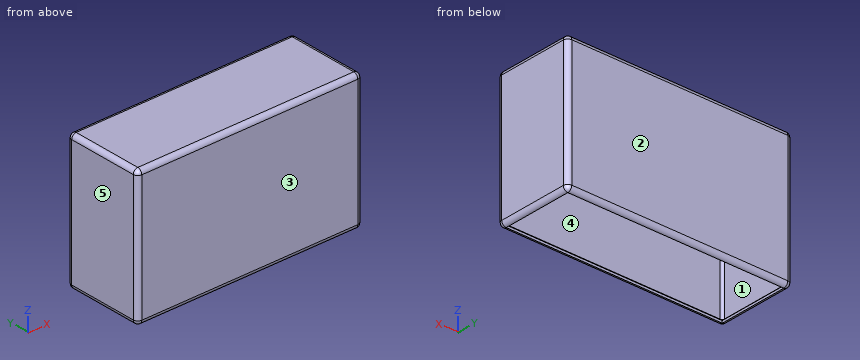
```python
from build123d import *

# Parameters (mm, degrees)
F0_W     = 254
F0_H     = 152.4
F1_DEPTH = 88.9
F2_R     = 5.08
F3_R     = 5.08
F4_R     = 5.08
F5_T     = -2.54


# Not quite as in the source:
# - a shell that OpenCascade refuses in one call is made with other operations: the cavity is built on its own and cut out


with BuildPart() as f1:
    # F0 (on Front) → F1 (new body)
    with BuildSketch(Plane.XZ):
        with Locations((-5.4093236282, -1.1136829853)):
            Rectangle(F0_W, F0_H)
    extrude(amount=F1_DEPTH)

    # F2
    f2_edges = [f1.edges().sort_by_distance(p)[0] for p in [
        (121.590676, -88.9, -1.113683),
        (121.590676, 0, -1.113683),
    ]]
    fillet(f2_edges, radius=F2_R)

    # F3
    f3_edges = [f1.edges().sort_by_distance(p)[0] for p in [
        (-7.949324, -88.9, 75.086317),
        (-7.949324, -88.9, -77.313683),
    ]]
    fillet(f3_edges, radius=F3_R)

    # F4
    f4_edges = [f1.edges().sort_by_distance(p)[0] for p in [
        (-132.409324, 0, -1.113683),
        (-132.409324, -88.9, -1.113683),
    ]]
    fillet(f4_edges, radius=F4_R)

    # F5: a shell. OpenCascade refuses it in one call, so the cavity is built on its own and cut out:
    # the body offset inwards by the wall thickness, plus a prism from it out through each open face.
    f5_core = offset(f1.part, amount=F5_T, mode=Mode.PRIVATE)
    f5_exits = [f5_core.faces().sort_by_distance(p)[0] for p in [
        (-5.409324, -44.45, -74.773683),
    ]]
    add(f5_core, mode=Mode.SUBTRACT)
    extrude(f5_exits, amount=-F5_T, mode=Mode.SUBTRACT)


solid = f1.part
```
Could you check a few things on this model? Use its own coordinates, in mm. Face numbers are marked on the shaded views. A direction names the side the tool comes from. Coordinates: 2 decimals unless noted, no trailing zeros. Order: outer loops, then holes, each group sorted by start corner. A loop starts at its lowest first (then second) coordinate and runs counter-clockwise, first axis right, second up. Notation, with made-up numbers: M 23,-33 L 62,-33 A20 cw 62,-27 Z; hole C 79.25,68.25 d5. An arc over 180 degrees is marked long. Use a Markdown table: item, result. Add a question column.
Q1. Which directions (+Z, -Z, +X, -X, +Y, -Y) give clear straight access to the entire face, cutting with the end or side of a thin tool? Please do the marked faces 1 and 2.
Q2. If I drill on L1, parallel to X at y = -12, z = 61; L2, parallel to Y at x = 3, z = -59; L3, parallel to Z at x = -84.5, y = -64, over which ranges is the centre line in solid material (lowest first)?
Q3. I want a section at A-A on z = -56. List the corners of the cut face in (x, y) for me.
Q4. I want a section at B-B on y = -80. List the corners of the cut face in (x, z) for me.
Q5. I want a section at C-C on x = 100. List the corners of the cut face in (y, z) for me.
Q6. We'd pull the mould along Y, two halves only. Please class the marked faces 3, 4 and 5: pulls with the +Y half, pulls with the -Y half, needs draft (parallel to the pull), parting line crosses it, or undercut.
Q7. I'm going to push flat-ended pins straight in: pin 1 (12 mm diameter, centred on x = -102.5, y = -65, fed in from -Z); pin 2 (0.8 mm diameter, centred on y = -54, z = -76, fed in from -X); pin 3 (2 mm diameter, centred on x = 40.5, z = -76.5, fed in from +Y). Where does each tip first touch, or does it pass through?
Checked values:
| question | item | result |
|---|---|---|
| 1 | face 1 | none |
| 1 | face 2 | +Z, -Z, +X, -X, +Y |
| 2 | L1 | -132.41 to -129.87, 119.05 to 121.59 |
| 2 | L2 | -88.9 to -86.36, -2.54 to 0 |
| 2 | L3 | 72.55 to 75.09 |
| 3 | outline | M -132.41,-83.82 A5.08 ccw -127.33,-88.9 L 116.51,-88.9 A5.08 ccw 121.59,-83.82 L 121.59,-5.08 A5.08 ccw 116.51,0 L -127.33,0 A5.08 ccw -132.41,-5.08 Z; hole M -129.87,-83.82 A2.54 ccw -127.33,-86.36 L 116.51,-86.36 A2.54 ccw 119.05,-83.82 L 119.05,-5.08 A2.54 ccw 116.51,-2.54 L -127.33,-2.54 A2.54 ccw -129.87,-5.08 Z |
| 4 | outline | M -132.41,-72.23 A5.08 ccw -127.33,-77.31 L -127.33,-74.77 A2.54 cw -129.87,-72.23 L -129.87,70.01 A2.54 cw -127.33,72.55 L 116.51,72.55 A2.54 cw 119.05,70.01 L 119.05,-72.23 A2.54 cw 116.51,-74.77 L 116.51,-77.31 A5.08 ccw 121.59,-72.23 L 121.59,70.01 A5.08 ccw 116.51,75.09 L -127.33,75.09 A5.08 ccw -132.41,70.01 Z |
| 5 | outline | M -88.9,-72.23 A5.08 ccw -83.82,-77.31 L -83.82,-74.77 A2.54 cw -86.36,-72.23 L -86.36,70.01 A2.54 cw -83.82,72.55 L -5.08,72.55 A2.54 cw -2.54,70.01 L -2.54,-72.23 A2.54 cw -5.08,-74.77 L -5.08,-77.31 A5.08 ccw 0,-72.23 L 0,70.01 A5.08 ccw -5.08,75.09 L -83.82,75.09 A5.08 ccw -88.9,70.01 Z |
| 6 | face 3 | pulls with the -Y half |
| 6 | face 4 | undercut |
| 6 | face 5 | needs draft |
| 7 | pin 1 | z = 72.55 |
| 7 | pin 2 | x = -131.13 |
| 7 | pin 3 | y = -1.19 |
